Autodesk Inventor part; units mm, degrees
ref_plane "Start Plane" through (0, 0, 0) normal (0, 0, 1) x (1, 0, 0)
ref_plane "End Plane" through (0, 0, 940) normal (0, 0, 1) x (1, 0, 0)
ref_plane "YZ Plane" through (0, 0, 0) normal (1, 0, 0) x (0, 1, 0)
ref_plane "Start Plane" through (0, 0, 0) normal (0, 0, 1) x (1, 0, 0)
ref_plane "End Plane" through (0, 0, 940) normal (0, 0, 1) x (1, 0, 0)
sketch "Sketch" plane through (0, 0, 0) normal (0, 0, 1) x (1, 0, 0)
  line L0 (-20, -24) -> (-20, 24)
  line L1 (-14, 30) -> (14, 30)
  line L2 (20, 24) -> (20, -24)
  line L3 (14, -30) -> (-14, -30)
  arc A0 (-20, -24) -> (-14, -30) centre (-14, -24) ccw
  arc A1 (20, 24) -> (14, 30) centre (14, 24) ccw
  arc A2 (-14, 30) -> (-20, 24) centre (-14, 24) ccw
  arc A3 (14, -30) -> (20, -24) centre (14, -24) ccw
  arc A4 (-14, 27) -> (-17, 24) centre (-14, 24) ccw
  line L4 (-14, 27) -> (14, 27)
  arc A5 (17, 24) -> (14, 27) centre (14, 24) ccw
  line L5 (17, 24) -> (17, -24)
  arc A6 (14, -27) -> (17, -24) centre (14, -24) ccw
  line L6 (14, -27) -> (-14, -27)
  arc A7 (-17, -24) -> (-14, -27) centre (-14, -24) ccw
  line L7 (-17, -24) -> (-17, 24)
  line L8 (0, 43.7397) -> (0, -43.7397) construction
  line L9 (-29.7397, 0) -> (29.7397, 0) construction
  dimension "d7" = 6
  dimension "d9" = 40
  dimension "d11" = 60
  dimension "d12" = 3
  dimension "d15" = 20
  dimension "d16" = 30
extrude "Body" add sketch "Sketch" along normal up to surface (940 mm away) from surface at 0
sketch "Sketch3" plane through (0, 0, 0) normal (0, 0, 1) x (1, 0, 0)
  line L0 (0, 0) -> (10, 0)
ref_plane "Work Plane3" through (0, 0, 0) normal (0, -1, 0) x (1, 0, 0)
sketch "Sketch4" plane through (0, 0, 0) normal (0, -1, 0) x (1, 0, 0)
  line L0 (-2, 0) -> (12, 0)
  line L1 (-2, 940) -> (12, 940)
  dimension "d18" = 940
equation "\"d7\" = G_IR"
equation "\"d9\" = G_W"
equation "\"d11\" = G_H"
equation "\"d12\" = G_T"
equation "\"d15\" = 0.5 * d9"
equation "\"d16\" = 0.5 * d11"
equation "\"d3\" = G_L"
equation "\"G_W\" = 40"
equation "\"G_H\" = 60"
equation "\"G_T\" = 3"
equation "\"G_IR\" = 6"
equation "\"G_L\" = d18"
equation "\"G_OFFSET_START\" = 0"
equation "\"G_OFFSET_END\" = 0"
properties part number "ISO 10799-2 - 60x40x3 - 940" material "Steel, Mild"
CAD build for the part. Positions are in the model's coordinates, mm. A direction names the side the tool comes from. Coordinates: 2 decimals unless noted, no trailing zeros. Loops run counter-clockwise (first coordinate to the right, second up) from the corner with the lowest first, then second, coordinate; pieces in that order, holes last. Notation, with made-up numbers: (-11.75, 80) - (-0.75, 80) arc R29 cw to (-0.75, 110) - close; hole circle Ø9 at (43.5, -29.75). An arc over 180 degrees is marked (long way). Write item = value, one per line. Start each with the question number.
Q1. Cut at A-A, the plane x = 6. List the corners of the cut face in (y, z).
Q2. Which spindle directions (+Z, -Z, +X, -X, +Y, -Y) get a long thin tool onto all of the face, cutting with end or side? Do faces 4 (the flat face through (0, 27, 463)), 5 (the flat face through (20, 0, 463)). Say none if no direction does.
Q3. Pull direction Y, two halves, no side cores. Call faces 1 (the flat face through (-17, 0, 463)), 2 (the flat face through (-18, 0, 940)), 3 (the flat face through (0, 30, 463)): pulls with the +Y half, pulls with the -Y half, needs draft (parallel to the pull), parting line crosses it, or undercut.
Q4. Cut at B-B, the plane y = -3.5. List the corners of the cut face in (x, z), then the cut area to 3 significant figures.
Q5. Drill centre lines: L1, parallel to X at y = 0, z = 820; L2, parallel to Y at x = -12.5, z = 666; L3, parallel to Y at x = 16.5, z = 378. Where is each one in solid material? Low to high.
Q6. Cut at C-C, the plane z = 183. List the corners of the cut face in (x, y), then the cut area to 3 significant figures.
Computed:
q1.outline = (-30, 0) - (-27, 0) - (-27, 940) - (-30, 940) - close; (27, 0) - (30, 0) - (30, 940) - (27, 940) - close
q2.face_4 = +Z, -Z
q2.face_5 = +Z, -Z, +X, +Y, -Y
q3.face_1 = undercut
q3.face_2 = needs draft
q3.face_3 = pulls with the +Y half
q4.outline = (-20, 0) - (-17, 0) - (-17, 940) - (-20, 940) - close; (17, 0) - (20, 0) - (20, 940) - (17, 940) - close
q4.area = 5,640 mm²
q5.L1 = -20 to -17, 17 to 20
q5.L2 = -30 to -27, 27 to 30
q5.L3 = -29.45 to -25.66, 25.66 to 29.45
q6.outline = (-20, -24) arc R6 ccw to (-14, -30) - (14, -30) arc R6 ccw to (20, -24) - (20, 24) arc R6 ccw to (14, 30) - (-14, 30) arc R6 ccw to (-20, 24) - close; hole (-17, -24) arc R3 ccw to (-14, -27) - (14, -27) arc R3 ccw to (17, -24) - (17, 24) arc R3 ccw to (14, 27) - (-14, 27) arc R3 ccw to (-17, 24) - close
q6.area = 541 mm²
